Verification items for the finished model (mm, model axes). A direction names the side the tool comes from. Give positions to 0.01 mm unless a question says otherwise; leave off trailing zeros. Write each loop counter-clockwise with the first axis right and the second up, starting at its lowest first coordinate (ties: lowest second). Pieces come first, ordered by that corner, then holes. Notation, with made-up numbers: M 88.5,-33.75 L 115.5,-33.75 A23 ccw 115.5,3.25 Z; hole C 74.25,79 d10. An arc over 180 degrees is marked long. Answer as a JSON object with one key per item and string values.
```python
from build123d import *

# Parameters (mm, degrees)
SKETCH1_W               = 22
SKETCH1_H               = 15
BOSS_EXTRUDE1_DEPTH     = 5
SKETCH2_W               = 3
SKETCH2_H               = 15
SKETCH2_H_2             = 14.97636143
BOSS_EXTRUDE2_DEPTH     = 5
CUT_EXTRUDE2_DEPTH      = 22.656407828
CUT_EXTRUDE2_DEPTH_BACK = 22.656407828
SKETCH4_R               = 1.5
FILLET1_R               = 8
FILLET3_RADIUS          = 1.5
FILLET3_LENGTH          = 14.97636143
FILLET4_RADIUS          = 1.5
FILLET4_LENGTH          = 15


with BuildPart() as part:
    # Sketch1 → Boss-Extrude1 (new body)
    with BuildSketch(Plane.XY):
        with Locations((-11, -7.5)):
            Rectangle(SKETCH1_W, SKETCH1_H)
    extrude(amount=BOSS_EXTRUDE1_DEPTH)

    # Sketch2 → Boss-Extrude2 (add)
    with BuildSketch(Plane.XY.offset(5)):
        with Locations((-8.5, -7.5)):
            Rectangle(SKETCH2_W, SKETCH2_H)
        with Locations((-13.5, -7.511819285)):
            Rectangle(SKETCH2_W, SKETCH2_H_2)
    extrude(amount=BOSS_EXTRUDE2_DEPTH)

    # Sketch4 → Cut-Extrude2 (cut, two sides: drawn at the far end of the back side and taken through both)
    with BuildSketch(Plane(origin=(-12, 0, 0), x_dir=(0, 0, -1), z_dir=(1, 0, 0)).offset(-CUT_EXTRUDE2_DEPTH_BACK)):
        with Locations(Location((-7.041389116, -7.762480296, 0), (0, 0, 270))):
            Circle(SKETCH4_R)
    extrude(amount=CUT_EXTRUDE2_DEPTH + CUT_EXTRUDE2_DEPTH_BACK, mode=Mode.SUBTRACT)

    # Fillet1
    # the kernel refuses this fillet: 8 mm, written as the material it takes off along each edge
    with BuildSketch(Plane(origin=(-22, 18.540496218, 5), x_dir=(1, 0, 0), z_dir=(0, -1, 0))) as fillet1_piece_1_section:
        with BuildLine():
            CenterArc((7.416198487, -8), FILLET1_R, 90, 67.975687163)
            Line((0, -5), (0, 0))
            Line((0, 0), (7.416198487, 0))
        make_face()
    fillet1_piece_1 = extrude(amount=52.080992435, mode=Mode.PRIVATE)
    fillet1_piece_1 = split(fillet1_piece_1, bisect_by=Plane(origin=(-22, -0.02363857, 5), z_dir=(0, 1, 0)), keep=Keep.TOP, mode=Mode.PRIVATE)
    add(fillet1_piece_1, mode=Mode.SUBTRACT)
    with BuildSketch(Plane(origin=(-22, 18.540496218, 5), x_dir=(1, 0, 0), z_dir=(0, -1, 0))) as fillet1_piece_2_section:
        with BuildLine():
            CenterArc((7.416198487, -8), FILLET1_R, 90, 67.975687163)
            Line((0, -5), (0, 0))
            Line((0, 0), (7.416198487, 0))
        make_face()
    fillet1_piece_2 = extrude(amount=52.080992435, mode=Mode.PRIVATE)
    fillet1_piece_2 = split(fillet1_piece_2, bisect_by=Plane(origin=(-15, 18.540496218, 5), z_dir=(-1, 0, 0)), keep=Keep.TOP, mode=Mode.PRIVATE)
    add(fillet1_piece_2, mode=Mode.SUBTRACT)
    with BuildSketch(Plane(origin=(0, -34.843134833, 5), x_dir=(0, 0, -1), z_dir=(0, 1, 0))) as fillet1_piece_3:
        with BuildLine():
            CenterArc((7.937253933, 8), FILLET1_R, 187.180755781, 82.819244219)
            Line((0, 7), (0, 0))
            Line((0, 0), (7.937253933, 0))
        make_face()
    extrude(amount=54.686269666, mode=Mode.SUBTRACT)

    # Fillet3: full round fillet: the end face becomes a half cylinder, R = half its width
    fillet3_face = Plane((-13.5, -7.511819285, 10), x_dir=(0, -1, 0), z_dir=(0, 0, 1))  # on the end face: x along it, z out of the body
    fillet3_slab = fillet3_face.offset(-FILLET3_RADIUS / 2) * Box(FILLET3_LENGTH, 2 * FILLET3_RADIUS, FILLET3_RADIUS, mode=Mode.PRIVATE)  # the body's end, R deep
    fillet3_round = Plane((-13.5, -7.511819285, 8.5), x_dir=(0, 0, 1), z_dir=(0, -1, 0)) * Cylinder(FILLET3_RADIUS, FILLET3_LENGTH, mode=Mode.PRIVATE)  # its axis R under the face
    add(fillet3_slab - fillet3_round, mode=Mode.SUBTRACT)

    # Fillet4: full round fillet: the end face becomes a half cylinder, R = half its width
    fillet4_face = Plane((-8.5, -7.5, 10), x_dir=(0, -1, 0), z_dir=(0, 0, 1))  # on the end face: x along it, z out of the body
    fillet4_slab = fillet4_face.offset(-FILLET4_RADIUS / 2) * Box(FILLET4_LENGTH, 2 * FILLET4_RADIUS, FILLET4_RADIUS, mode=Mode.PRIVATE)  # the body's end, R deep
    fillet4_round = Plane((-8.5, -7.5, 8.5), x_dir=(0, 0, 1), z_dir=(0, -1, 0)) * Cylinder(FILLET4_RADIUS, FILLET4_LENGTH, mode=Mode.PRIVATE)  # its axis R under the face
    add(fillet4_slab - fillet4_round, mode=Mode.SUBTRACT)


solid = part.part
```
1) Section check D-D on y = -5.75. Record the boundary of the cut face in (x, z), and give its area (3 significant figures).
Completed:
{"outline": "M -22,0 L -0.56,0 A8 ccw -7,5 L -7,8.5 A1.5 ccw -10,8.5 L -10,5 L -12,5 L -12,8.5 A1.5 ccw -15,8.5 L -15,4.99 A8 ccw Z", "area": "115 mm2"}
2) Go/stop test with flat-tipped pins: pin 1 (4 mm diameter, centred on y = -7.76, z = 7.04, fed in from +X); pin 2 (6 mm diameter, centred on y = -13.5, z = 4, fed in from -X); pin 3 (3 mm diameter, centred on y = -9, z = 4.5, fed in from -X); pin 4 (5 mm diameter, centred on x = -16.5, z = 6.5, fed in from +Y). Record where each tip stops, or that it passes through.
Completed:
{"pin 1": "stops at x = -7", "pin 2": "stops at x = -21.51", "pin 3": "stops at x = -19.88", "pin 4": "stops at y = 0"}
3) Section check A-A on y = -7.75. Record the boundary of the cut face in (x, z), and give its area (3 significant figures).
Completed:
{"outline": "M -22,0 L -0.56,0 A8 ccw -7,5 L -7,5.54 L -10,5.54 L -10,5 L -12,5 L -12,5.54 L -15,5.54 L -15,4.99 A8 ccw Z; M -15,8.54 L -12,8.54 A1.5 ccw Z; M -10,8.54 L -7,8.54 A1.5 ccw Z", "area": "97.1 mm2"}
4) Section check C-C on z = 9.25. Record the boundary of the cut face in (x, y).
Completed:
{"outline": "M -14.8,-15 L -12.2,-15 L -12.2,-0.02 L -14.8,-0.02 Z; M -9.8,-15 L -7.2,-15 L -7.2,0 L -9.8,0 Z"}
5) Release check for a two-part mould opening along Y. For faces 6 (the face through (-7, -7.6, 5.2)), 7 (the face through (-11, -15, 4)), 8 (the face through (-8.521, -9.148, 7.616)) record: pulls with the +Y half, pulls with the -Y half, needs draft (parallel to the pull), parting line crosses it, or undercut.
Completed:
{"face 6": "needs draft", "face 7": "pulls with the -Y half", "face 8": "undercut"}
6) Access from +Z, -Z, +X, -X, +Y, -Y to the whole of each face (thin tool, end or side, straight path). Record for faces 1 (the face through (-12, -7.6, 5.2)), 2 (the face through (-3.142, -7.605, 3.419)), 3 (the face through (-15, -7.6, 5.2)), 4 (the face through (-13, -0.024, 7)), 5 (the face through (-11, -7, 0)).
Completed:
{"face 1": "+Z, +Y, -Y", "face 2": "+Z, +X, +Y, -Y", "face 3": "+Z, -X, +Y, -Y", "face 4": "+Z, -X, +Y", "face 5": "-Z, +X, -X, +Y, -Y"}
7) Thickness scan on L1, parallel to X at y = -13.75, z = 6; L2, parallel to Y at x = -12.5, z = 6.75; L3, parallel to X at y = -4.75, z = 9.5. Record the ranges inside material, lowest first.
Completed:
{"L1": "x = -15 to -12, -10 to -7", "L2": "y = -15 to -9.23, -6.29 to -0.02", "L3": "x = -14.62 to -12.38, -9.62 to -7.38"}
